CAD build for the part. Positions are in the model's coordinates, mm. A direction names the side the tool comes from. Coordinates: 2 decimals unless noted, no trailing zeros. Loops run counter-clockwise (first coordinate to the right, second up) from the corner with the lowest first, then second, coordinate; pieces in that order, holes last. Notation, with made-up numbers: (53.25, 68) -> (95.25, 68) arc R24 cw to (95.25, 101) -> close; hole circle Ø3 at (-11, -37.75). An arc over 180 degrees is marked (long way). Return JSON: item names as keys, results as strings. Group by question number.
(1) Flat gauge pin, fed straight in: pin 1 Ø1 at (y, z) = (-2, 0) entering from -X. Where does the tip first touch, or does it go through?
(2) Saw through at B-B on x = -9.5. Write the cut outline in (y, z), then the cut area to 3 significant figures.
(3) Probe L1, parallel to Z at x = 35, y = 1.5; L2, parallel to Z at x = 27, y = 0. List the from-to ranges inside material, lowest first.
(4) Tool access for faces 5 (the face through (-34, -3.65, -0.04)), 6 (the face through (-40, 0, -3)), 7 (the face through (5.97, -0.54, -2.44)): list every direction of +Z, -Z, +X, -X, +Y, -Y with a clear straight run to the whole face (end or side of a thin tool).
(5) Mould opens along X. For faces 1 (the face through (-34, 3.6, -0.7)), 2 (the face through (-39, -4, 0)), 3 (the face through (-48, 0, 0)), 4 (the face through (-46, 0, 0)) say: pulls with the +X half, pulls with the -X half, needs draft (parallel to the pull), parting line crosses it, or undercut.
(6) Saw through at A-A on z = 0. Write the cut outline in (x, y), then the cut area to 3 significant figures.
Solid Edge part; units mm, degrees
sketch "Sketch1" plane through (0, 0, 0) normal (1, 0, 0) x (0, 1, 0)
  circle A0 centre (0, 0) radius 2.5
extrude "Protrusion1" add sketch "Sketch1" along normal blind 44
sketch "Sketch2" plane through (0, 0, 0) normal (1, 0, 0) x (0, 1, 0)
  circle A0 centre (0, 0) radius 2.5
extrude "ExtrudedProtrusion_2" add sketch "Sketch2" against normal blind 34
sketch "Sketch3" plane through (0, 0, 0) normal (0, 0, 1) x (1, 0, 0)
  line L0 (-44, -4) -> (-34, -4)
  line L1 (-34, -4) -> (-34, 4)
  line L2 (-34, 4) -> (-44, 4)
  arc A0 (-44, 4) -> (-44, -4) centre (-44, 0) ccw
  circle A1 centre (-44, 0) radius 2
extrude "ExtrudedProtrusion_3" add sketch "Sketch3" along normal mid plane 6
fillet "Round_1" radius 1 1 edges at (-34, -2.5, 0)
cosmetic_thread "Thread_1" thread depth 14
Geometry results:
{
 "1": {"pin 1": "x = -47.71"},
 "2": {"outline": "circle Ø5 at (0, 0)", "area": "19.6 mm²"},
 "3": {"L1": "-2 to 2", "L2": "-2.5 to 2.5"},
 "4": {"face 5": "+X, -Y", "face 6": "-Z, +X, -X, +Y, -Y", "face 7": "+X"},
 "5": {"face 1": "pulls with the +X half", "face 2": "needs draft", "face 3": "pulls with the -X half", "face 4": "undercut"},
 "6": {"outline": "(-44, -4) -> (-34, -4) -> (-34, -3.5) arc R1 cw to (-33, -2.5) -> (44, -2.5) -> (44, 2.5) -> (-33, 2.5) arc R1 cw to (-34, 3.5) -> (-34, 4) -> (-44, 4) arc R4 ccw to start; hole circle Ø4 at (-44, 0)", "area": "483 mm²"}
}
